Check sheet for the drawn part. Datum: minimum x, y, z corner. Units: mm. A direction names the side the tool comes from. Coordinates: 2 decimals unless noted, no trailing zeros. Loops run counter-clockwise (first coordinate to the right, second up) from the corner with the lowest first, then second, coordinate; pieces in that order, holes last. Notation, with made-up numbers: (-37, 32.25) -> (19, 32.25) arc R22 cw to (19, 44.25) -> close; hole circle Ø8 at (81, 21.5). An arc over 180 degrees is marked (long way). Use CSV: the item, a comma, the result in double quotes. Start each with the question number.
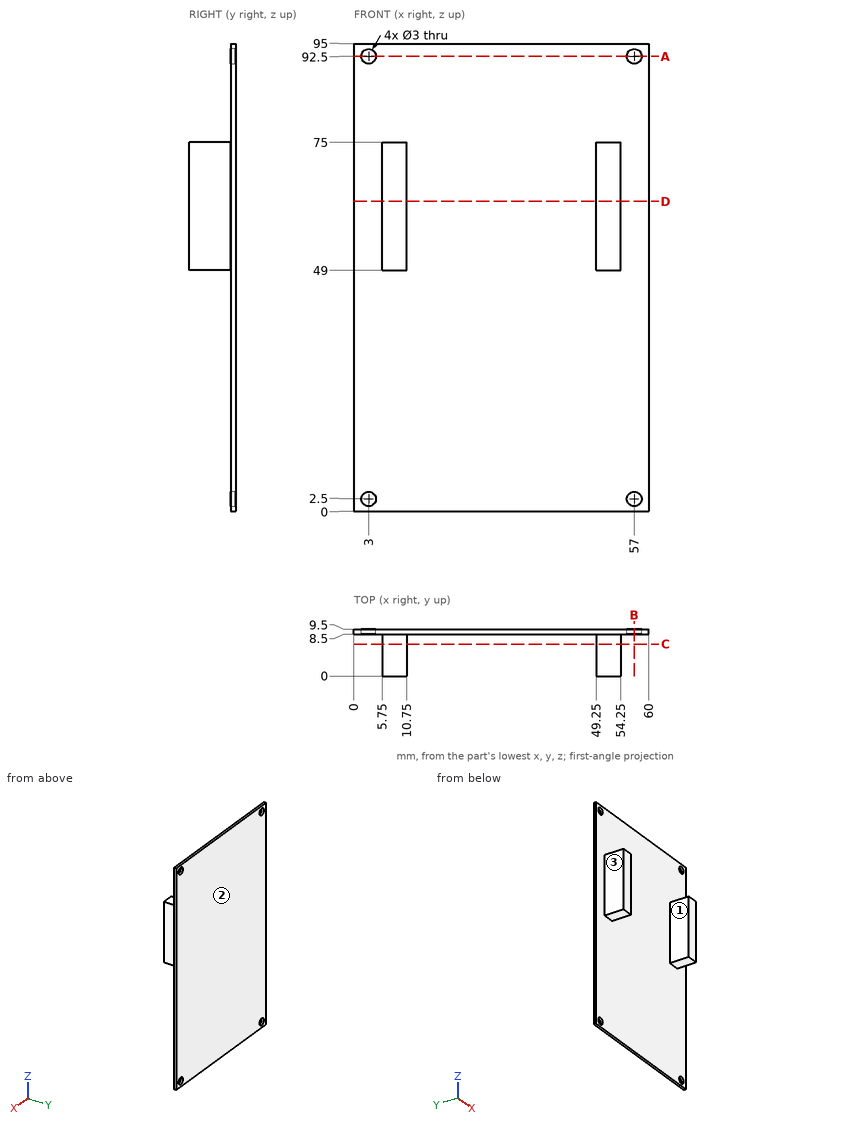
1. Scan lines: line 1 (X direction, y = 9.15, z = 2.5); line 2 (X direction, y = 6, z = 62); line 3 (Y direction, x = 47.5, z = 90). Record each from-to range of solid material in increasing order.
2. Cross-section at C-C, the plane y = 6.5. Record the boundary of the cut face in (x, z), plus the area to 3 significant figures.
3. Set-up check for the marked faces 1, 2 and 3: record each of +Z, -Z, +X, -X, +Y, -Y from which the full face is reachable in a straight line by a thin tool's end or side.
4. Cross-section at B-B, the plane x = 57. Record the boundary of the cut face in (y, z).
5. Cross-section at D-D, the plane z = 63. Record the boundary of the cut face in (x, y).
6. Cross-section at A-A, the plane z = 92.5. Record the boundary of the cut face in (x, y).
7. Depth check by flat-ended pin: pin 1 (1.5 mm diameter, centred on x = 51.5, y = 4, fed in from -Z); pin 2 (5 mm diameter, centred on x = 57, z = 92.5, fed in from -Y); pin 3 (4 mm diameter, centred on x = 50.5, y = 3, fed in from +Z); pin 4 (2.5 mm diameter, centred on x = 3, z = 92.5, fed in from +Y) (1 decimal). Enter the tip coordinate at first touch or a pass-through.
Solution:
1,line 1,"x = 0 to 1.5, 4.5 to 55.5, 58.5 to 60"
1,line 2,"x = 5.75 to 10.75, 49.25 to 54.25"
1,line 3,"y = 8.5 to 9.5"
2,outline,"(5.75, 49) -> (10.75, 49) -> (10.75, 75) -> (5.75, 75) -> close; (49.25, 49) -> (54.25, 49) -> (54.25, 75) -> (49.25, 75) -> close"
2,area,"260 mm2"
3,face 1,"+Z, -Z, -Y"
3,face 2,"+Z, -Z, +X, -X, +Y"
3,face 3,"+Z, -Z, -X, -Y"
4,outline,"(8.5, 0) -> (9.5, 0) -> (9.5, 1) -> (8.5, 1) -> close; (8.5, 4) -> (9.5, 4) -> (9.5, 91) -> (8.5, 91) -> close; (8.5, 94) -> (9.5, 94) -> (9.5, 95) -> (8.5, 95) -> close"
5,outline,"(0, 8.5) -> (5.75, 8.5) -> (5.75, 0) -> (10.75, 0) -> (10.75, 8.5) -> (49.25, 8.5) -> (49.25, 0) -> (54.25, 0) -> (54.25, 8.5) -> (60, 8.5) -> (60, 9.5) -> (0, 9.5) -> close"
6,outline,"(0, 8.5) -> (1.5, 8.5) -> (1.5, 9.5) -> (0, 9.5) -> close; (4.5, 8.5) -> (55.5, 8.5) -> (55.5, 9.5) -> (4.5, 9.5) -> close; (58.5, 8.5) -> (60, 8.5) -> (60, 9.5) -> (58.5, 9.5) -> close"
7,pin 1,"stops at z = 49"
7,pin 2,"stops at y = 8.5"
7,pin 3,"stops at z = 75"
7,pin 4,"passes through"
